Autodesk Inventor part; units mm, degrees
ref_plane "YZ Plane" through (0, 0, 0) normal (1, 0, 0) x (0, 1, 0)
ref_plane "XZ Plane" through (0, 0, 0) normal (0, 1, 0) x (-1, 0, 0)
ref_plane "XY Plane" through (0, 0, 0) normal (0, 0, 1) x (1, 0, 0)
sketch "Sketch2" plane through (0, 0, 0) normal (0, 0, 1) x (1, 0, 0)
  circle A0 centre (0, 0) radius 25
  line L0 (-17.0079, 22.5) -> (27.1684, 22.5)
  point P0 (10.8972, 22.5)
  point P1 (-10.8972, 22.5)
  dimension "d4" = 50
  dimension "d5" = 22.5
extrude "Extrusion2" add sketch "Sketch2" along normal blind 27 contours A0 L0 picked at (1.1654, 4.7055)
sketch "Sketch3" plane through (-10.8972, 22.5, 0) normal (0, 1, 0) x (1, 0, 0)
  circle A0 centre (10.8972, -13.5) radius 2.875
  line L0 (0, 0) -> (0, -27)
  line L1 (21.7945, 0) -> (21.7945, -27)
  line L2 (21.7945, 0) -> (0, 0)
  point P0 (10.8972, 0)
  dimension "d8" = 5.75
  dimension "d9" = 10.8972
  dimension "d10" = 21.7945
  dimension "d11" = 27
  dimension "d12" = 13.5
extrude "Extrusion3" cut sketch "Sketch3" against normal blind 15
sketch "Sketch4" plane through (0, 0, 27) normal (0, 0, 1) x (1, 0, 0)
  line L0 (6.2132, -15) -> (15, -6.2132)
  line L1 (-6.2132, -15) -> (6.2132, -15)
  line L2 (-15, -6.2132) -> (-6.2132, -15)
  line L3 (-15, 6.2132) -> (-15, -6.2132)
  line L4 (-6.2132, 15) -> (-15, 6.2132)
  line L5 (6.2132, 15) -> (-6.2132, 15)
  line L6 (15, 6.2132) -> (6.2132, 15)
  line L7 (15, -6.2132) -> (15, 6.2132)
  line L8 (-6.1884, 14.94) -> (6.1884, 14.94)
  line L9 (6.1884, 14.94) -> (14.94, 6.1884)
  line L10 (14.94, 6.1884) -> (14.94, -6.1884)
  line L11 (14.94, -6.1884) -> (6.1884, -14.94)
  line L12 (6.1884, -14.94) -> (-6.1884, -14.94)
  line L13 (-6.1884, -14.94) -> (-14.94, -6.1884)
  line L14 (-14.94, -6.1884) -> (-14.94, 6.1884)
  line L15 (-14.94, 6.1884) -> (-6.1884, 14.94)
  point P0 (0, 0)
  point P1 (0, 0)
  dimension "d47" = 29.88
  dimension "d48" = 14.94
  dimension "d49" = 14.94
  dimension "d50" = 29.88
extrude "Extrusion4" cut sketch "Sketch4" against normal blind 20 contours L8 L9 L10 L11 L12 L13 L14 L15
sketch "Sketch6" plane through (0, 0, 27) normal (0, 0, 1) x (1, 0, 0)
  line L0 (-15.1, 6.2546) -> (-6.2546, 15.1)
  line L1 (-15.1, -6.2546) -> (-15.1, 6.2546)
  line L2 (-6.2546, -15.1) -> (-15.1, -6.2546)
  line L3 (6.2546, -15.1) -> (-6.2546, -15.1)
  line L4 (15.1, -6.2546) -> (6.2546, -15.1)
  line L5 (15.1, 6.2546) -> (15.1, -6.2546)
  line L6 (6.2546, 15.1) -> (15.1, 6.2546)
  line L7 (-6.2546, 15.1) -> (6.2546, 15.1)
  line L8 (0, 0) -> (33.369, 0)
  circle A0 centre (0, 0) radius 20
  circle A1 centre (20, 0) radius 2.9
  circle A2 centre (-20, 0) radius 2.9
  dimension "d20" = 40
  dimension "d21" = 5.8
  dimension "d24" = 360
extrude "Extrusion6" cut sketch "Sketch6" against normal blind 7 contours A1 A0 L8 | L8 A0 A1 | A0 A1 L8 | L8 A1 A0 | A2 A0 | A0 A2
sketch "Sketch7" plane through (0, 0, 0) normal (0, 0, -1) x (-1, 0, 0)
  line L0 (0, 0) -> (41.4197, 0)
  circle A0 centre (20, 0) radius 2.9
  circle A1 centre (20, 0) radius 2.9
  circle A2 centre (14.1421, 14.1421) radius 2.9
  circle A3 centre (0, 20) radius 2.9
  circle A4 centre (-14.1421, 14.1421) radius 2.9
  circle A5 centre (-20, 0) radius 2.9
  circle A6 centre (-14.1421, -14.1421) radius 2.9
  circle A7 centre (0, -20) radius 2.9
  circle A8 centre (14.1421, -14.1421) radius 2.9
  dimension "d30" = 360
extrude "Extrusion7" cut sketch "Sketch7" against normal blind 10 contours A0 L0 | L0 A0 | A2 | A4 | A5 | A6 | A7 | A8
sketch "Sketch8" plane through (0, 0, 7) normal (0, 0, 1) x (1, 0, 0)
  line L0 (-15.1, 6.2546) -> (-6.2546, 15.1)
  line L1 (-15.1, -6.2546) -> (-15.1, 6.2546)
  line L2 (-6.2546, -15.1) -> (-15.1, -6.2546)
  line L3 (6.2546, -15.1) -> (-6.2546, -15.1)
  line L4 (15.1, -6.2546) -> (6.2546, -15.1)
  line L5 (15.1, 6.2546) -> (15.1, -6.2546)
  line L6 (6.2546, 15.1) -> (15.1, 6.2546)
  line L7 (-6.2546, 15.1) -> (6.2546, 15.1)
  line L8 (3.7693, 9.1) -> (9.1, 3.7693)
  line L9 (9.1, 3.7693) -> (9.1, -3.7693)
  line L10 (9.1, -3.7693) -> (3.7693, -9.1)
  line L11 (3.7693, -9.1) -> (-3.7693, -9.1)
  line L12 (-3.7693, -9.1) -> (-9.1, -3.7693)
  line L13 (-9.1, -3.7693) -> (-9.1, 3.7693)
  line L14 (-9.1, 3.7693) -> (-3.7693, 9.1)
  line L15 (-3.7693, 9.1) -> (3.7693, 9.1)
  point P0 (0, 0)
  dimension "d34" = 6
extrude "Extrusion8" cut sketch "Sketch8" against normal through all contours L8 L9 L10 L11 L12 L13 L14 L15
chamfer "Chamfer1" distance 0.2 angle 45 8 edges at (9.1, 0, 0) (6.4347, 6.4347, 0) (0, 9.1, 0) (-6.4347, 6.4347, 0) (-9.1, 0, 0) (-6.4347, -6.4347, 0) (0, -9.1, 0) (6.4347, -6.4347, 0)
chamfer "Chamfer2" distance 0.2 angle 45 9 edges at (17.0421, 14.1421, 0) (-11.2421, 14.1421, 0) (-17.1, 0, 0) (-11.2421, -14.1421, 0) (2.9, -20, 0) (17.0421, -14.1421, 0) (22.9, 0, 0) (-22.9, 0, 27) (17.1, 0, 27)
chamfer "Chamfer3" distance 0.2 angle 45 4 edges at (0, -25, 0) (0, 22.5, 0) (0, -25, 27) (0, 22.5, 27)
chamfer "Chamfer4" distance 0.2 angle 45 8 edges at (0, 14.94, 27) (10.5642, 10.5642, 27) (14.94, 0, 27) (10.5642, -10.5642, 27) (0, -14.94, 27) (-10.5642, -10.5642, 27) (-14.94, 0, 27) (-10.5642, 10.5642, 27)
equation "\"d9\" = 0.5 * d10"
equation "\"d12\" = 0.5 * d11"
equation "\"d50\" = d47"
properties part number "spool_center"
Check sheet for the modelled part. Datum: model origin and axes. Units: mm. A direction names the side the tool comes from. Round coordinates to 2 decimals unless told otherwise and drop trailing zeros. Loops run counter-clockwise (first coordinate to the right, second up) from the corner with the lowest first, then second, coordinate; pieces in that order, holes last. Notation, with made-up numbers: (30.25, 6.5) -> (89.25, 6.5) arc R24 cw to (89.25, 35.5) -> close; hole circle Ø4 at (48.5, 26). An arc over 180 degrees is marked (long way). Put each result on its own line as item: value. Start each with the question number.
1. Section check A-A (x = 0). Give the number of separate pieces and of enclosed holes in the cut face, plus the area to 3 significant figures.
2. Access from +Z, -Z, +X, -X, +Y, -Y to the whole of each face (thin tool, end or side, straight path). Record for faces 1 (the face through (-9.1, 0, 4)), 2 (the face through (0, 14.94, 17)), 3 (the face through (0, -20, 10)).
3. Draft check along X on faces 4 (the face through (0, -11, 0)), 5 (the face through (14, -14, 10)). Enter one of: +X half, -X half, draft (parallel to the pull), parting line (faces both ways), or undercut.
4. Scan lines: probe 1 along X at (y, z) = (-1.5, 22.25); probe 2 along X at (y, z) = (-16.5, 8.5); probe 3 along Y at (x, z) = (-2, 7.75). Record each from-to range of solid material in increasing order.
5. Gauge pin test, flat ends, axial feed: pin 1 (10 mm diameter, centred on y = 8.5, z = 16.5, fed in from +X); pin 2 (6.5 mm diameter, centred on x = -20, y = 0, fed in from -Z); pin 3 (4 mm diameter, centred on x = 16.5, z = 19.5, fed in from +Y); pin 4 (3 mm diameter, centred on y = 10, z = 18, fed in from +X). Record the tip position at first contact, or that the pin passes through.
6. Section check C-C (z = 11.25). Enter the section's corners in (x, y).
Findings:
1. separate pieces: 3
1. enclosed holes: 0
1. area: 456 mm^2
2. face 1: +Z, -Z
2. face 2: +Z
2. face 3: -Z
3. face 4: draft
3. face 5: undercut
4. probe 1: x = -24.95 to -22.48, -17.52 to -14.94, 14.94 to 17.52, 22.48 to 24.95
4. probe 2: x = -18.78 to -15.83, -12.45 to 12.45, 15.83 to 18.78
4. probe 3: y = -24.92 to -22.1, -17.9 to -14.94, 14.94 to 22.5
5. pin 1: stops at x = 24.75
5. pin 2: stops at z = 0
5. pin 3: stops at y = 20.37
5. pin 4: stops at x = 23.51
6. outline: (-14.94, -6.19) -> (-14.94, 6.19) -> (-6.19, 14.94) -> (-1.79, 14.94) -> (-1.79, 22.5) -> (-10.9, 22.5) arc R25 ccw (long way) to (10.9, 22.5) -> (1.79, 22.5) -> (1.79, 14.94) -> (6.19, 14.94) -> (14.94, 6.19) -> (14.94, -6.19) -> (6.19, -14.94) -> (-6.19, -14.94) -> close
